Input: part model. Units: mm. Frame: model coordinates. Face numbers are marked on the shaded views. Round coordinates to 2 decimals unless told otherwise and drop trailing zeros. Loops run counter-clockwise (first coordinate to the right, second up) from the corner with the lowest first, then second, coordinate; pieces in that order, holes last.
(1) Cut plane A-A, the plane y = 6.75. Output: boundary loops of the cut face in (x, z).
(2) Cut plane D-D, the plane y = -1. Output: boundary loops of the cut face in (x, z), and give its area (3 significant figures).
(3) Draft query along Z for the marked faces 1, 2, 3 and 4. Return one class per face: released by +Z, released by -Z, zero draft, split by the parting line, or undercut.
(4) Cut plane B-B, the plane x = 0. Output: boundary loops of the cut face in (y, z).
(5) First-contact query: pin 1 Ø3.5 at (x, z) = (1.5, -11.5) entering from +Y; pin 2 Ø6 at (y, z) = (8.5, -8.5) entering from -X; pin 3 Ø1 at (y, z) = (9.5, -5.5) entering from +X. Flat tips, straight axial feed; report the tip coordinate or a pass-through.
(6) Cut plane C-C, the plane z = 0. Output: boundary loops of the cut face in (x, y).
(7) Line query: line 1 (X direction, y = 2, z = 0); line 2 (Z direction, x = 0, y = 9.25); line 3 (Y direction, x = 1, z = -13.5). Output: solid intervals per line, ascending.
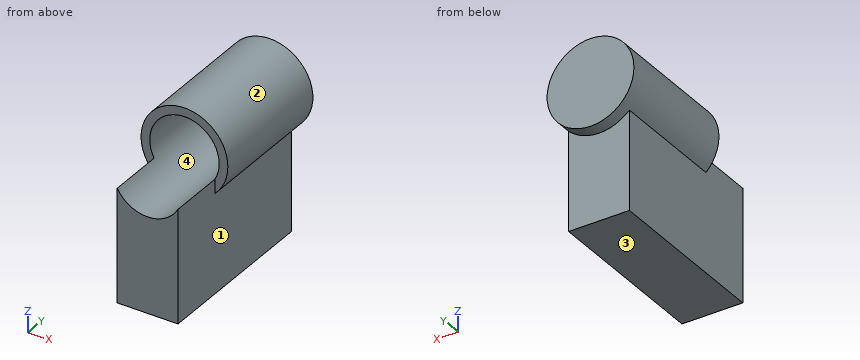
Autodesk Inventor part; units mm, degrees
ref_plane "YZ Plane" through (0, 0, 0) normal (1, 0, 0) x (0, 1, 0)
ref_plane "XZ Plane" through (0, 0, 0) normal (0, 1, 0) x (-1, 0, 0)
ref_plane "XY Plane" through (0, 0, 0) normal (0, 0, 1) x (1, 0, 0)
sketch "スケッチ1" plane through (0, 0, 0) normal (0, 1, 0) x (-1, 0, 0)
  circle A0 centre (0, 0) radius 5
  dimension "d0" = 10
extrude "押し出し1" add sketch "スケッチ1" along normal blind 15
sketch "スケッチ2" plane through (0, 15, 0) normal (0, 1, 0) x (1, 0, 0)
  line L0 (0, 0) -> (0, 5)
  circle A0 centre (0, 0) radius 5
sketch "スケッチ3" plane through (0, 15, 0) normal (0, 1, 0) x (1, 0, 0)
  point P0 (0, 0)
sketch "スケッチ4" plane through (0, 0, 0) normal (0, -1, 0) x (1, 0, 0)
  line L0 (0, 0) -> (0, -5)
  circle A0 centre (0, 0) radius 5
ref_plane "作業平面1" through (0, 0, -5) normal (0, 0, -1) x (-1, 0, 0)
sketch "スケッチ5" plane through (0, 0, -5) normal (0, 0, -1) x (-1, 0, 0)
  line L0 (5, 15) -> (-5, 15)
  line L1 (0, 15) -> (0, 0)
sketch "スケッチ7" plane through (0, 0, 0) normal (0, -1, 0) x (1, 0, 0)
  circle A0 centre (0, 0) radius 4
  dimension "d3" = 8
sketch "スケッチ8" plane through (0, 0, -5) normal (0, 0, -1) x (-1, 0, 0)
  line L0 (3.5, 13.5) -> (-3.5, 13.5)
  line L1 (-3.5, 13.5) -> (-3.5, -6.5)
  line L2 (-3.5, -6.5) -> (3.5, -6.5)
  line L3 (3.5, -6.5) -> (3.5, 13.5)
  line L4 (5, 15) -> (-5, 15)
  line L5 (0, 15) -> (0, 0)
  line L6 (5, 0) -> (5, 15)
  line L7 (5, 15) -> (-5, 15)
  line L8 (5, 0) -> (-5, 0)
  dimension "d6" = 1.5
  dimension "d7" = 7
  dimension "d8" = 20
extrude "押し出し4" add sketch "スケッチ8" against normal blind 5 contours L3 L8 L5 L0 | L5 L8 L1 L0 | L3 L2 L1 L8
extrude "押し出し5" cut sketch "スケッチ7" along normal mid plane 26
extrude "押し出し6" add sketch "スケッチ8" along normal blind 10 contours L3 L8 L5 L0 | L5 L8 L1 L0 | L3 L2 L1 L8
properties part number "tale outer"
Reported:
1. outline: (-3.5, -15) - (3.5, -15) - (3.5, -3.57) arc R5 ccw (long way) to (-3.5, -3.57) - close; hole circle Ø8 at (0, 0)
2. outline: (-3.5, -15) - (3.5, -15) - (3.5, -1.94) arc R4 cw to (-3.5, -1.94) - close
2. area: 81.2 mm2
3. face 1: zero draft
3. face 2: split by the parting line
3. face 3: released by -Z
3. face 4: undercut
4. outline: (-6.5, -15) - (13.5, -15) - (13.5, -5) - (15, -5) - (15, 5) - (0, 5) - (0, 4) - (13, 4) - (13, -4) - (-6.5, -4) - close
5. pin 1: stops at y = 13.5
5. pin 2: stops at x = -3.5
5. pin 3: stops at x = 3.5
6. outline: (-5, 0) - (-4, 0) - (-4, 13) - (4, 13) - (4, 0) - (5, 0) - (5, 15) - (-5, 15) - close
7. line 1: x = -5 to -4, 4 to 5
7. line 2: z = -15 to -4, 4 to 5
7. line 3: y = -6.5 to 13.5
